Check sheet for the modelled part. Datum: model origin and axes. Units: mm. Face numbers are marked on the shaded views. A direction names the side the tool comes from. Coordinates: 2 decimals unless noted, no trailing zeros. Order: outer loops, then holes, each group sorted by start corner. A loop starts at its lowest first (then second) coordinate and runs counter-clockwise, first axis right, second up. Notation, with made-up numbers: (-22.75, 40.25) -> (-2.75, 40.25) arc R21 ccw to (-2.75, 57.25) -> close; hole circle Ø4 at (30.5, -18.5). An arc over 180 degrees is marked (long way). Put each result on its own line as item: value. Start each with the question number.
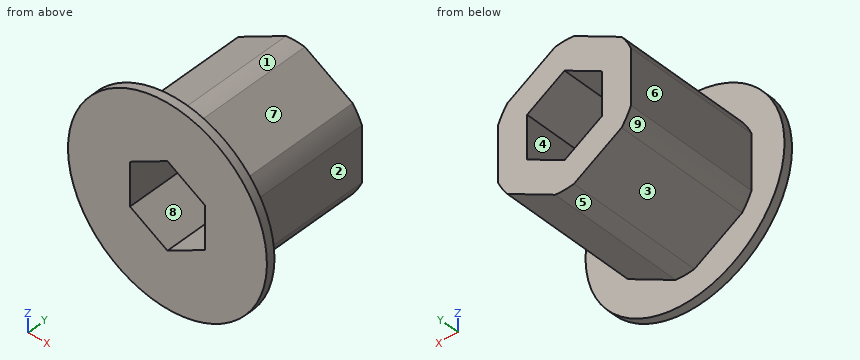
```python
from build123d import *

# Parameters (mm, degrees)
SKETCH1_R           = 9.5
BOSS_EXTRUDE1_DEPTH = 0.79375
BOSS_EXTRUDE2_DEPTH = 12.7


with BuildPart() as part:
    # Sketch1 → Boss-Extrude1 (new body)
    with BuildSketch(Plane(origin=(0, 0, 0), x_dir=(1, 0, 0), z_dir=(0, 1, 0))):
        with Locations(Location((0, 0, 0), (0, 0, 270))):
            Circle(SKETCH1_R)
        Polygon((0, 4.128054425), (-3.575, 2.064027212), (-3.575, -2.064027212), (0, -4.128054425), (3.575, -2.064027212), (3.575, 2.064027212), align=None, mode=Mode.SUBTRACT)
    extrude(amount=BOSS_EXTRUDE1_DEPTH)

    # Sketch2 → Boss-Extrude2 (add)
    with BuildSketch(Plane(origin=(0, 0.79375, 0), x_dir=(1, 0, 0), z_dir=(0, 1, 0))):
        with BuildLine():
            ThreePointArc((0.893039494, 6.816751826), (0, 6.875), (-0.893039494, 6.816751826))
            Line((-0.893039494, 6.816751826), (-5.456960506, 4.181770802))
            ThreePointArc((-5.456960506, 4.181770802), (-5.953924651, 3.4375), (-6.35, 2.634981025))
            Line((-6.35, 2.634981025), (-6.35, -2.634981025))
            ThreePointArc((-6.35, -2.634981025), (-5.953924651, -3.4375), (-5.456960506, -4.181770802))
            Line((-5.456960506, -4.181770802), (-0.893039494, -6.816751826))
            ThreePointArc((-0.893039494, -6.816751826), (0, -6.875), (0.893039494, -6.816751826))
            Line((0.893039494, -6.816751826), (5.456960506, -4.181770802))
            ThreePointArc((5.456960506, -4.181770802), (5.953924651, -3.4375), (6.35, -2.634981025))
            Line((6.35, -2.634981025), (6.35, 2.634981025))
            ThreePointArc((6.35, 2.634981025), (5.953924651, 3.4375), (5.456960506, 4.181770802))
            Line((5.456960506, 4.181770802), (0.893039494, 6.816751826))
        make_face()
        Polygon((-3.575, 2.064027212), (0, 4.128054425), (3.575, 2.064027212), (3.575, -2.064027212), (0, -4.128054425), (-3.575, -2.064027212), align=None, mode=Mode.SUBTRACT)
    extrude(amount=BOSS_EXTRUDE2_DEPTH)


solid = part.part
```
1) Access from +Z, -Z, +X, -X, +Y, -Y to the whole of each face (thin tool, end or side, straight path). Record for the marked faces 1, 2, 3, 4 and 5.
2) Sectioned sample at B-B (y = 2). Record the boundary of the cut face in (x, z) (3 decimals).
3) Scan lines: line 1 along X through (y, z) = (2, 1) (3 decimals); line 2 along X through (y, z) = (4.75, 3.25); line 3 along Y through (x, z) = (4.75, -8). Record each from-to range of solid material in increasing order. Write a range as [from, to].
4) Sectioned sample at C-C (x = -2.75). Record the boundary of the cut face in (y, z), plus the area to 3 significant figures.
5) Gauge pin test, flat ends, axial feed: pin 1 (3 mm diameter, centred on x = 2.5, y = 1.5, fed in from -Z); pin 2 (2 mm diameter, centred on y = 7, z = 1, fed in from +X); pin 3 (5 mm diameter, centred on x = -6.5, y = 9.5, fed in from -Z). Record the tip position at first contact, or that the pin passes through.
6) Sectioned sample at A-A (z = 0). Record the boundary of the cut face in (x, y) (3 decimals).
7) Mould release check, pull along Z, two halves, no side actions. Record for the marked faces 6, 7, 8 and 9: +Z half, -Z half, draft (parallel to the pull), parting line (faces both ways), or undercut.
8) Sectioned sample at D-D (x = 5.75). Record the boundary of the cut face in (y, z).
Entries:
1. face 1: +Z, +Y
1. face 2: +Z, -Z, +X, +Y
1. face 3: -Z, -X, +Y
1. face 4: +Y, -Y
1. face 5: -Z, +Y
2. outline: (-6.35, -2.635) arc R6.875 ccw to (-5.457, -4.182) -> (-0.893, -6.817) arc R6.875 ccw to (0.893, -6.817) -> (5.457, -4.182) arc R6.875 ccw to (6.35, -2.635) -> (6.35, 2.635) arc R6.875 ccw to (5.457, 4.182) -> (0.893, 6.817) arc R6.875 ccw to (-0.893, 6.817) -> (-5.457, 4.182) arc R6.875 ccw to (-6.35, 2.635) -> close; hole (-3.575, -2.064) -> (0, -4.128) -> (3.575, -2.064) -> (3.575, 2.064) -> (0, 4.128) -> (-3.575, 2.064) -> close
3. line 1: x = [-6.35, -3.575], [3.575, 6.35]
3. line 2: x = [-6.06, -1.52], [1.52, 6.06]
3. line 3: y = [0, 0.79]
4. outline: (0, -9.09) -> (0.79, -9.09) -> (0.79, -5.74) -> (13.49, -5.74) -> (13.49, -2.54) -> (0, -2.54) -> close; (0, 2.54) -> (13.49, 2.54) -> (13.49, 5.74) -> (0.79, 5.74) -> (0.79, 9.09) -> (0, 9.09) -> close
4. area: 91.8 mm2
5. pin 1: stops at z = -9.43
5. pin 2: stops at x = 6.35
5. pin 3: stops at z = -5.02
6. outline: (-9.5, 0) -> (-3.575, 0) -> (-3.575, 13.494) -> (-6.35, 13.494) -> (-6.35, 0.794) -> (-9.5, 0.794) -> close; (3.575, 0) -> (9.5, 0) -> (9.5, 0.794) -> (6.35, 0.794) -> (6.35, 13.494) -> (3.575, 13.494) -> close
7. face 6: draft
7. face 7: +Z half
7. face 8: undercut
7. face 9: -Z half
8. outline: (0, -7.56) -> (0.79, -7.56) -> (0.79, -3.77) -> (13.49, -3.77) -> (13.49, 3.77) -> (0.79, 3.77) -> (0.79, 7.56) -> (0, 7.56) -> close
